Answer from the drawing. Dimensions are ordinates in mm from the lowest x, y and z of the part. A direction names the side the tool comes from. Coordinates: 2 decimals unless noted, no trailing zeros. Order: outer loops, then holes, each group sorted by start corner. A loop starts at its lowest first (then second) coordinate and runs counter-clockwise, first axis right, second up. Notation, with made-up numbers: (-13.75, 30.5) - (-3.75, 30.5) arc R7 ccw to (-3.75, 34.5) - close; hole circle Ø3 at (68.25, 34). An arc over 180 degrees is marked (long way). Answer as a JSON object with one key per item and string values. Group by question number.
1) A tool of negligible diameter and unlimited length cuts with its end or side. For the marked faces 1, 2, 3, 4 and 5, from which of +Z, -Z, +X, -X, +Y, -Y can it reach the whole face along a straight path? Write none if from no direction.
2) Find the intervals of material crossed by line 1 along Y through (x, z) = (2, 1.35); line 2 along Y through (x, z) = (10, 3.5), in increasing order.
3) Section D-D (x = 2) is taken. Give the vertices of the cut face in (y, z), plus the area to 3 significant figures.
4) Each of these flat-tipped pins is pushed along its axis until it touches: P1, Ø2, axis at y = 14.5, z = 5, coming from the +X side; P2, Ø3, axis at y = 11, z = 9, coming from the +X side; P3, Ø3, axis at x = 15.5, z = 8, coming from the +Y side. Where does it stop, or does it pass through?
5) Section C-C (y = 17.2) is taken. Give the vertices of the cut face in (x, z), plus the area to 3 significant figures.
6) Section A-A (y = 9.75) is taken. Give the vertices of the cut face in (x, z).
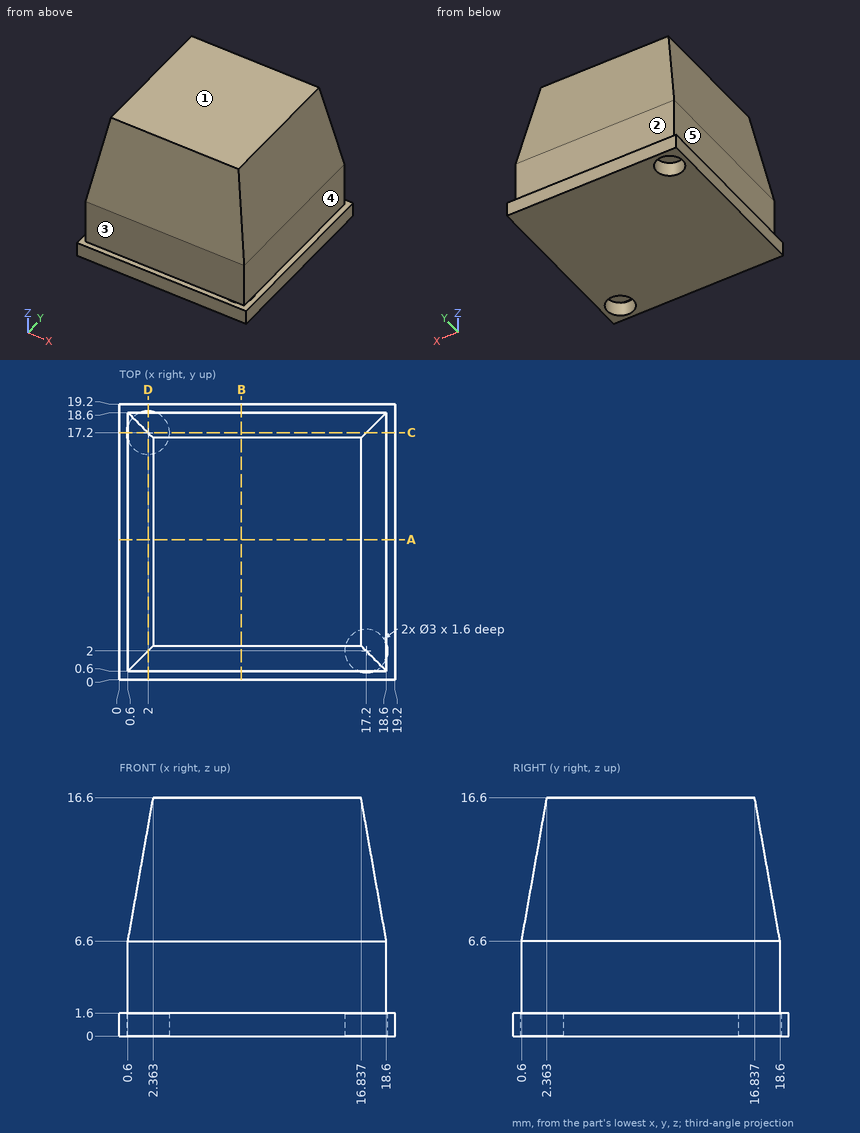
Report:
{
 "1": {"face 1": "+Z, +X, -X, +Y, -Y", "face 2": "+Z, +X, -X, +Y", "face 3": "+Z, +X, -X, -Y", "face 4": "+Z, +X, +Y, -Y", "face 5": "+Z, -X, +Y, -Y"},
 "2": {"line 1": "y = 0 to 15.7, 18.7 to 19.2", "line 2": "y = 0.6 to 18.6"},
 "3": {"outline": "(0, 0) - (15.7, 0) - (15.7, 1.6) - (18.6, 1.6) - (18.6, 6.6) - (17.2, 14.54) - (2, 14.54) - (0.6, 6.6) - (0.6, 1.6) - (0, 1.6) - close; (18.7, 0) - (19.2, 0) - (19.2, 1.6) - (18.7, 1.6) - close", "area": "248 mm²"},
 "4": {"P1": "stops at x = 18.6", "P2": "stops at x = 18.44", "P3": "stops at y = 18.6"},
 "5": {"outline": "(0, 0) - (0.5, 0) - (0.5, 1.6) - (0, 1.6) - close; (0.6, 1.6) - (3.5, 1.6) - (3.5, 0) - (19.2, 0) - (19.2, 1.6) - (18.6, 1.6) - (18.6, 6.6) - (17.2, 14.54) - (2, 14.54) - (0.6, 6.6) - close", "area": "248 mm²"},
 "6": {"outline": "(0, 0) - (19.2, 0) - (19.2, 1.6) - (18.6, 1.6) - (18.6, 6.6) - (16.84, 16.6) - (2.36, 16.6) - (0.6, 6.6) - (0.6, 1.6) - (0, 1.6) - close"}
}
